```python
from build123d import *

# Parameters (mm, degrees)
PAD_DEPTH       = 20
POCKET_DEPTH    = 12
SKETCH002_R     = 2.9
SKETCH003_R     = 1.9
SKETCH004_R     = 2.9
SKETCH005_R     = 1.9
POCKET001_DEPTH = 24.001
POCKET002_DEPTH = 3
SKETCH012_R     = 3.55
SKETCH013_R     = 1.5
CHAMFER_SIZE    = 0.5
CHAMFER001_SIZE = 1


with BuildPart() as part:
    # Sketch → Pad (new body)
    with BuildSketch(Plane.XY):
        with BuildLine():
            ThreePointArc((35, 0), (47, 12), (35, 24))
            Line((35, 24), (4, 24))
            ThreePointArc((4, 24), (1.171573, 22.828427), (0, 20))
            Line((0, 20), (0, 16.5))
            Line((0, 16.5), (29.040134, 16.5))
            ThreePointArc((40.955468, 16.52), (34.989761, 21.299991), (29.040134, 16.5))
            Line((40.955468, 16.52), (42.255468, 16.52))
            ThreePointArc((42.255468, 13.88), (43.575468, 15.2), (42.255468, 16.52))
            Line((40.955468, 13.88), (42.255468, 13.88))
            ThreePointArc((29.040134, 13.9), (34.989761, 9.100009), (40.955468, 13.88))
            Line((24.140134, 9), (29.040134, 13.9))
            Line((8.3, 9), (24.140134, 9))
            Line((8.3, 1.5), (8.3, 9))
            ThreePointArc((8.3, 1.5), (8.73934, 0.43934), (9.8, 0))
            Line((35, 0), (9.8, 0))
        make_face()
    extrude(amount=PAD_DEPTH)

    # Sketch001 → Pocket (cut)
    with BuildSketch(Plane.XZ.offset(-4)):
        with BuildLine():
            Line((17.2, 10), (17.2, 4))
            Line((17.2, 4), (35.1, 4))
            Line((35.1, 4), (35.1, 20))
            Line((35.1, 20), (0, 20))
            Line((0, 20), (0, 4))
            Line((0, 4), (11.4, 4))
            Line((11.4, 4), (11.4, 10))
            ThreePointArc((17.2, 10), (14.3, 12.9), (11.4, 10))
        make_face()
    extrude(amount=-POCKET_DEPTH, mode=Mode.SUBTRACT)

    # Sketch002 → AdditiveLoft section 0
    with BuildSketch(Plane.XZ.offset(-9)):
        with Locations((14.3, 10)):
            Circle(SKETCH002_R)
    # Sketch003 → AdditiveLoft section 1
    with BuildSketch(Plane.XZ.offset(-10.75)):
        with Locations((14.3, 10)):
            Circle(SKETCH003_R)
    loft()

    # Sketch004 → AdditiveLoft001 section 0
    with BuildSketch(Plane.XZ.offset(-16.5)):
        with Locations((14.3, 10)):
            Circle(SKETCH004_R)
    # Sketch005 → AdditiveLoft001 section 1
    with BuildSketch(Plane.XZ.offset(-14.75)):
        with Locations((14.3, 10)):
            Circle(SKETCH005_R)
    loft()

    # Sketch006 → AdditiveLoft002 section 0
    with BuildSketch(Plane.XZ.offset(-9)):
        with BuildLine():
            ThreePointArc((11.4, 6), (14.3, 5.059352), (17.2, 6))
            Line((17.2, 6), (17.2, 3.5))
            ThreePointArc((11.4, 3.5), (14.3, 2.882416), (17.2, 3.5))
            Line((11.4, 6), (11.4, 3.5))
        make_face()
    # Sketch007 → AdditiveLoft002 section 1
    with BuildSketch(Plane.XZ.offset(-9.5)):
        with BuildLine():
            ThreePointArc((12.7, 5), (14.3, 4.750238), (15.9, 5))
            Line((15.9, 5), (15.9, 4.5))
            ThreePointArc((12.7, 4.5), (14.3, 4.271999), (15.9, 4.5))
            Line((12.7, 5), (12.7, 4.5))
        make_face()
    loft()

    # Sketch008 → AdditiveLoft003 section 0
    with BuildSketch(Plane.XZ.offset(-16.5)):
        with BuildLine():
            ThreePointArc((11.4, 6), (14.3, 5.059352), (17.2, 6))
            Line((17.2, 6), (17.2, 3.5))
            ThreePointArc((11.4, 3.5), (14.3, 2.882416), (17.2, 3.5))
            Line((11.4, 6), (11.4, 3.5))
        make_face()
    # Sketch009 → AdditiveLoft003 section 1
    with BuildSketch(Plane.XZ.offset(-16)):
        with BuildLine():
            ThreePointArc((12.7, 5), (14.3, 4.750238), (15.9, 5))
            Line((15.9, 5), (15.9, 4.5))
            ThreePointArc((12.7, 4.5), (14.3, 4.271999), (15.9, 4.5))
            Line((12.7, 5), (12.7, 4.5))
        make_face()
    loft()

    # Sketch010 → Pocket001 (cut, through all)
    with BuildSketch(Plane.XZ):
        with BuildLine():
            ThreePointArc((13.133274, 11.166726), (14.3, 8.35), (15.466726, 11.166726))
            Line((15.466726, 11.166726), (14.8, 11.833452))
            Line((13.8, 11.833452), (14.8, 11.833452))
            Line((13.133274, 11.166726), (13.8, 11.833452))
        make_face()
    extrude(amount=-POCKET001_DEPTH, mode=Mode.SUBTRACT)

    # Sketch011 → Pocket002 (cut)
    with BuildSketch(Plane.XZ.offset(-24)):
        Polygon((11.55, 11.587713), (11.55, 8.412287), (14.3, 6.824574), (17.05, 8.412287), (17.05, 11.587713), (14.3, 13.175426), align=None)
    extrude(amount=POCKET002_DEPTH, mode=Mode.SUBTRACT)

    # Sketch012 → SubtractiveLoft section 0
    with BuildSketch(Plane.XZ):
        with Locations((14.3, 10)):
            Circle(SKETCH012_R)
    # Sketch013 → SubtractiveLoft section 1
    with BuildSketch(Plane.XZ.offset(-2.05)):
        with Locations((14.3, 10)):
            Circle(SKETCH013_R)
    loft(mode=Mode.SUBTRACT)

    # Chamfer
    chamfer_edges = [part.edges().sort_by_distance(p)[0] for p in [
        (15.675, 24, 7.61843),
        (17.05, 24, 10),
        (15.675, 24, 12.38157),
        (12.925, 24, 12.38157),
        (11.55, 24, 10),
        (12.925, 24, 7.61843),
    ]]
    chamfer(chamfer_edges, length=CHAMFER_SIZE)

    # Chamfer001
    chamfer001_edges = [part.edges().sort_by_distance(p)[0] for p in [
        (21.7, 4, 20),
        (35.1, 6.55041, 20),
        (14.520067, 16.5, 20),
    ]]
    chamfer(chamfer001_edges, length=CHAMFER001_SIZE)


solid = part.part
```
Here's how the part is built. I have some questions about the finished solid (model axes, mm). A direction names the side the tool comes from. Give positions to 0.01 mm unless a question says otherwise; leave off trailing zeros. Write each loop counter-clockwise with the first axis right and the second up, starting at its lowest first coordinate (ties: lowest second). Pieces come first, ordered by that corner, then holes.
(1) Imagine slicing it at D-D, the plane y = 12. Write out the boundary of the cut face in (x, z).
Output values:
outline: (27.14, 0) - (29.81, 0) - (29.81, 4) - (27.14, 4) - close; (40.19, 0) - (47, 0) - (47, 20) - (40.19, 20) - close
(2) Imagine slicing it at C-C, the plane y = 6.5. Write out the boundary of the cut face in (x, z), and give its area (3 significant figures).
Output values:
outline: (8.3, 0) - (45.67, 0) - (45.67, 20) - (36.1, 20) - (35.1, 19) - (35.1, 4) - (17.2, 4) - (17.2, 10) arc R2.9 ccw to (11.4, 10) - (11.4, 4) - (8.3, 4) - close; hole (13.13, 11.17) arc R1.65 ccw (long way) to (15.47, 11.17) - (14.8, 11.83) - (13.8, 11.83) - close
area: 357 mm2
(3) If I drill on L1, parallel to Y at x = 29, z = 13; L2, parallel to X at y = 17.5, z = 10; L3, parallel to Y at x = 16, z = 1.75, over which ranges is the centre line in solid material (lowest first)?
Output values:
L1: y = 0 to 4, 16.5 to 24
L2: x = 0 to 12.65, 15.95 to 29.35, 40.65 to 45.67
L3: y = 0 to 9, 16.5 to 24
(4) Imagine slicing it at B-B, the plane y = 15.5. Write out the boundary of the cut face in (x, z), and give its area (3 significant figures).
Output values:
outline: circle Ø4.66 at (14.3, 10); (43.54, 0) - (46.48, 0) - (46.48, 20) - (43.54, 20) - close; hole (13.13, 11.17) arc R1.65 ccw (long way) to (15.47, 11.17) - (14.8, 11.83) - (13.8, 11.83) - close
area: 66.9 mm2
(5) On a 3-axis mill with a long thin cutter (end or side, diameter ignored), from which of +Z, -Z, +X, -X, +Y, -Y can I reach the whole of each face in a straight line? I mean faces 1 (the face through (14, 6, 11.833)), 2 (the face through (14, 9, 6)), 3 (the face through (22, 4, 12)), 4 (the face through (15.66, 22.27, 7.61)). Say none if no direction works.
Output values:
face 1: +Y, -Y
face 2: none
face 3: +Z
face 4: +Y
(6) Imagine slicing it at A-A, the plane x = 22. Write out the boundary of the cut face in (y, z), and give its area (3 significant figures).
Output values:
outline: (0, 0) - (9, 0) - (9, 4) - (4, 4) - (4, 19) - (3, 20) - (0, 20) - close; (16.5, 0) - (24, 0) - (24, 20) - (17.5, 20) - (16.5, 19) - close
area: 249 mm2
(7) Will these pins go through, and if not, where does the flat tip stop? pin 1 (2 mm diameter, centred on x = 14.3, z = 10, fed in from -Y); pin 2 (5.5 mm diameter, centred on y = 5.5, z = 5.5, fed in from -X); pin 3 (1.5 mm diameter, centred on y = 21.5, z = 2, fed in from +X); pin 4 (1.2 mm diameter, centred on y = 22.5, z = 10, fed in from +X).
Output values:
pin 1: passes through
pin 2: stops at x = 8.3
pin 3: stops at x = 43.21
pin 4: stops at x = 41.78
(8) Thinking about a two-plate mould opening in X: for faces 5 (the face through (10, 6, 4)), 6 (the face through (43.575, 15.171, 9.86)), 7 (the face through (8.3, 3.5, 7.6)), which applies, pulls with the +X half, pulls with the -X half, needs draft (parallel to the pull), parting line crosses it, or undercut?
Output values:
face 5: needs draft
face 6: undercut
face 7: pulls with the -X half
